Build history of the part. All positions in model axes, mm. Face numbers are marked on the shaded views. A direction names the side the tool comes from. Coordinates: 2 decimals unless noted, no trailing zeros. Loops run counter-clockwise (first coordinate to the right, second up) from the corner with the lowest first, then second, coordinate; pieces in that order, holes last.
Item 1: Drill centre lines: line 1 along X through (y, z) = (-5, 2.4); line 2 along X through (y, z) = (-6.5, 1.4); line 3 along X through (y, z) = (-8, 0.4). Where is each one in solid material? Low to high.
Item 2: Cut at C-C (y = -11.5). List the corners of the cut face in (x, z).
Item 3: Cut at B-B (x = -4.8). List the corners of the cut face in (y, z).
Item 4: Cut at D-D (z = 4.15). List the corners of the cut face in (x, y) (3 decimals).
Item 5: Mould opens along Y. For the marked faces 1, 2 and 3 say: released by +Y, released by -Y, zero draft, split by the parting line, or undercut.
Item 6: Cut at A-A (y = -6). List the corners of the cut face in (x, z).
Item 7: Flat gauge pins, fed straight in: pin 1 (3 mm diameter, centred on x = -4, y = -11, fed in from -Z); pin 2 (1.3 mm diameter, centred on x = 11, y = -5.5, fed in from +Z); pin 3 (2.5 mm diameter, centred on x = -4.8, y = -11, fed in from +Z). Where does each tip first touch, or does it go through?
Item 8: 3-axis set-ups, long thin cutter, end or side, ignore diameter. For the marked faces 4, 5 and 6: which of +Z, -Z, +X, -X, +Y, -Y reach the whole face in a straight line?
from build123d import *

# Parameters (mm, degrees)
ESBO_O1_R                = 1.375
RESSALTO_EXTRUS_O3_DEPTH = 4.5
ESBO_O7_R                = 1.625
CORTE_EXTRUS_O4_DEPTH    = 21.605917331
ESBO_O8_R                = 2.15
CORTE_EXTRUS_O5_DEPTH    = 2
ESBO_O9_R                = 2.9
CORTE_EXTRUS_O6_DEPTH    = 3.5


with BuildPart() as part:
    # Esboço1 → Ressalto-extrusão3 (new body)
    with BuildSketch(Plane.XY):
        with BuildLine():
            ThreePointArc((-7.794228634, -4.5), (-11.892304845, -3.401923789), (-12.990381057, -7.5))
            ThreePointArc((-12.990381057, -7.5), (0, -15), (12.990381057, -7.5))
            ThreePointArc((12.990381057, -7.5), (11.892304845, -3.401923789), (7.794228634, -4.5))
            ThreePointArc((7.794228634, -4.5), (0, -9), (-7.794228634, -4.5))
        make_face()
        with Locations((-10.392304845, -6)):
            Circle(ESBO_O1_R, mode=Mode.SUBTRACT)
        with Locations(Location((10.392304845, -6, 0), (0, 0, 180))):
            Circle(ESBO_O1_R, mode=Mode.SUBTRACT)
    extrude(amount=RESSALTO_EXTRUS_O3_DEPTH)

    # Esboço7 → Corte-extrusão4 (cut, through all)
    with BuildSketch(Plane.XY.offset(4.5)):
        with Locations((-4.8, -10.998181668)):
            Circle(ESBO_O7_R)
    extrude(amount=-CORTE_EXTRUS_O4_DEPTH, mode=Mode.SUBTRACT)

    # Esboço8 → Corte-extrusão5 (cut)
    with BuildSketch(Plane.XY.offset(4.5)):
        with Locations((-10.392304845, -6)):
            Circle(ESBO_O8_R)
        with Locations((10.392304845, -6)):
            Circle(ESBO_O8_R)
    extrude(amount=-CORTE_EXTRUS_O5_DEPTH, mode=Mode.SUBTRACT)

    # Esboço9 → Corte-extrusão6 (cut)
    with BuildSketch(Plane(origin=(0, 0, 0), x_dir=(-1, 0, 0), z_dir=(0, 0, -1))):
        with Locations((4.8, -10.998181668)):
            Circle(ESBO_O9_R)
    extrude(amount=-CORTE_EXTRUS_O6_DEPTH, mode=Mode.SUBTRACT)


solid = part.part
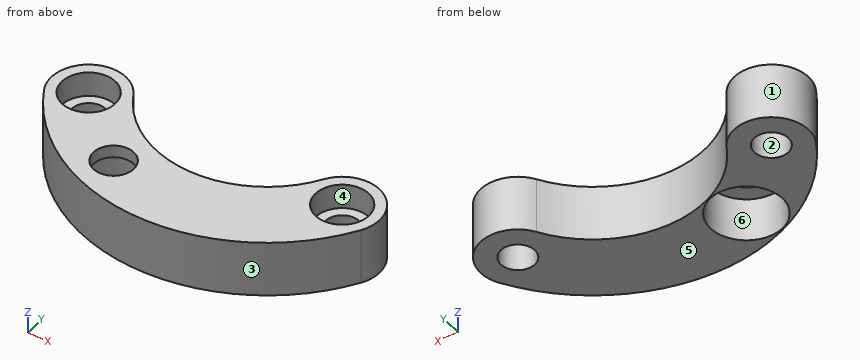
Filled sheet:
1. line 1: x = -13.22 to -11.34, -9.45 to -7.48, 7.48 to 9.45, 11.34 to 13.22
1. line 2: x = -13.35 to -11.67, -9.11 to -6.22, 6.22 to 9.11, 11.67 to 13.35
1. line 3: x = -12.69 to -4.12, 4.12 to 12.69
2. outline: (-9.63, 0) - (-7.66, 0) - (-7.66, 3.5) - (-6.35, 3.5) - (-6.35, 4.5) - (-9.63, 4.5) - close; (-3.25, 3.5) - (-1.94, 3.5) - (-1.94, 0) - (9.63, 0) - (9.63, 4.5) - (-3.25, 4.5) - close
3. outline: (-14.21, 0) - (-13.9, 0) - (-13.9, 3.5) - (-12.62, 3.5) - (-12.62, 4.5) - (-14.21, 4.5) - close; (-9.37, 3.5) - (-8.1, 3.5) - (-8.1, 0) - (-7.61, 0) - (-7.61, 4.5) - (-9.37, 4.5) - close
4. outline: (-12.99, -7.5) arc R15 ccw to (12.99, -7.5) arc R3 ccw to (7.794, -4.5) arc R9 cw to (-7.794, -4.5) arc R3 ccw to start; hole circle Ø4.3 at (-10.392, -6); hole circle Ø3.25 at (-4.8, -10.998); hole circle Ø4.3 at (10.392, -6)
5. face 1: split by the parting line
5. face 2: undercut
5. face 3: released by -Y
6. outline: (-13.39, 0) - (-11.77, 0) - (-11.77, 2.5) - (-12.54, 2.5) - (-12.54, 4.5) - (-13.39, 4.5) - close; (-9.02, 0) - (-6.71, 0) - (-6.71, 4.5) - (-8.24, 4.5) - (-8.24, 2.5) - (-9.02, 2.5) - close; (6.71, 0) - (9.02, 0) - (9.02, 2.5) - (8.24, 2.5) - (8.24, 4.5) - (6.71, 4.5) - close; (11.77, 0) - (13.39, 0) - (13.39, 4.5) - (12.54, 4.5) - (12.54, 2.5) - (11.77, 2.5) - close
7. pin 1: stops at z = 3.5
7. pin 2: stops at z = 2.5
7. pin 3: passes through
8. face 4: +Z
8. face 5: -Z, +X, -X, +Y, -Y
8. face 6: -Z
